```python
from build123d import *

# Parameters (mm, degrees)
BOSS_EXTRUDE1_DEPTH      = 20
BOSS_EXTRUDE1_DEPTH_BACK = 20
SKETCH1_W                = 15
SKETCH1_H                = 220
CUT_EXTRUDE1_REACH       = 193.638
SKETCH5_R                = 14.2875


with BuildPart() as part:
    # Sketch1 → Boss-Extrude1 (new, two sides: drawn at the far end of the back side and taken through both)
    with BuildSketch(Plane.ZY.offset(-BOSS_EXTRUDE1_DEPTH_BACK)):
        with Locations((-7.5, 80)):
            Rectangle(SKETCH1_W, SKETCH1_H)
    extrude(amount=BOSS_EXTRUDE1_DEPTH + BOSS_EXTRUDE1_DEPTH_BACK)

    # Sketch5 → Cut-Extrude1 (cut, up to next)
    with BuildSketch(Plane(origin=(0, 0, -15), x_dir=(-1, 0, 0), z_dir=(0, 0, -1)), mode=Mode.PRIVATE) as cut_extrude1_sk1:
        with Locations((0, 167.443589791)):
            Circle(SKETCH5_R)
    cut_extrude1_tool1 = extrude(cut_extrude1_sk1.sketch, amount=-CUT_EXTRUDE1_REACH, mode=Mode.PRIVATE) & part.part
    add(cut_extrude1_tool1.solids().sort_by_distance((0, 167.44359, -15))[0], mode=Mode.SUBTRACT)


solid = part.part
```
Check sheet for the modelled part. Datum: model origin and axes. Units: mm. Coordinates: 2 decimals unless noted, no trailing zeros. Order: outer loops, then holes, each group sorted by start corner. A loop starts at its lowest first (then second) coordinate and runs counter-clockwise, first axis right, second up. Notation, with made-up numbers: (68.25, 27) -> (105.25, 27) arc R16 ccw to (105.25, 44) -> close; hole circle Ø2 at (50, 2). An arc over 180 degrees is marked (long way). Write item = value, one per line. Start each with the question number.
1) Cross-section at B-B (z = -12.5). Enter the section's corners in (x, y) (1 decimal).
2) Material ranges on L1, parallel to Y at x = 0, z = -8.5; L2, parallel to Y at x = -6, z = -12.5; L3, parallel to X at y = 175.5, z = -13, recorded low to high.
3) Cross-section at C-C (x = 10.5). Enter the section's corners in (y, z), then the cut area to 3 significant figures.
4) Cross-section at A-A (x = 0). Enter the section's corners in (y, z), then the cut area to 3 significant figures.
5) Mould release check, pull along Y, two halves, no side actions. Record for faces 1 (the flat face through (0, 190, -8)), 2 (the flat face through (0, 78, 0)), 3 (the cylindrical face through (1.86, 181.61, -7.6)): +Y half, -Y half, draft (parallel to the pull), parting line (faces both ways), or undercut.
Ans:
q1.outline = (-20, -30) -> (20, -30) -> (20, 190) -> (-20, 190) -> close; hole circle Ø28.6 at (0, 167.4)
q2.L1 = -30 to 153.16, 181.73 to 190
q2.L2 = -30 to 154.48, 180.41 to 190
q2.L3 = -20 to -11.8, 11.8 to 20
q3.outline = (-30, -15) -> (157.75, -15) -> (157.75, 0) -> (-30, 0) -> close; (177.13, -15) -> (190, -15) -> (190, 0) -> (177.13, 0) -> close
q3.area = 3,010 mm²
q4.outline = (-30, -15) -> (153.16, -15) -> (153.16, 0) -> (-30, 0) -> close; (181.73, -15) -> (190, -15) -> (190, 0) -> (181.73, 0) -> close
q4.area = 2,870 mm²
q5.face_1 = +Y half
q5.face_2 = draft
q5.face_3 = undercut
